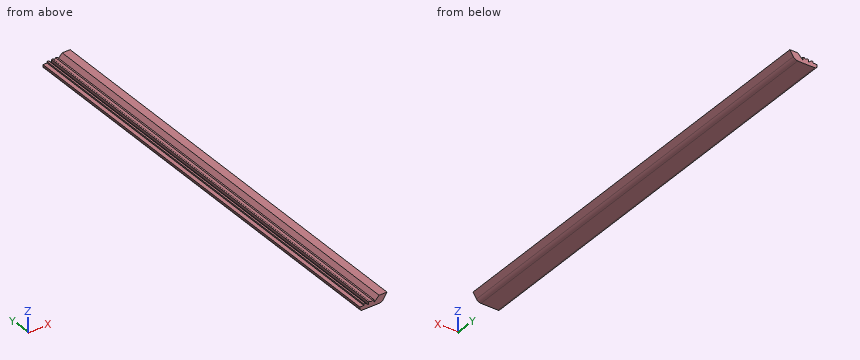
```python
from build123d import *

# Parameters (mm, degrees)
PAD_DEPTH    = 775
POCKET_DEPTH = 800


with BuildPart() as part:
    # Sketch → Pad (new body)
    with BuildSketch(Plane.XZ):
        with BuildLine():
            Line((14, -4), (-16, -4))
            ThreePointArc((-20, 0), (-18.828427, -2.828427), (-16, -4))
            Line((-20, 3), (-20, 0))
            Line((-13, 3), (-20, 3))
            Line((-13, 5.5), (-13, 3))
            Line((-10, 5.5), (-13, 5.5))
            Line((-10, 5.5), (-5, 1))
            Line((-5, 6), (-5, 1))
            Line((5, 6), (-5, 6))
            Line((5, 6), (5, 1))
            Line((14, 10), (5, 1))
            Line((28, 10), (14, 10))
            Line((21.78, 0.396373), (28, 10))
            ThreePointArc((14, -4), (18.428584, -2.754913), (21.78, 0.396373))
        make_face()
    extrude(amount=PAD_DEPTH)

    # Sketch001 (on Face16 of Pad) → Pocket (cut)
    with BuildSketch(Plane.XZ.offset(775)):
        with BuildLine():
            ThreePointArc((-2.51, 6.117451), (0, 4.67), (2.51, 6.117451))
            Line((-2.51, 6.117451), (2.51, 6.117451))
        make_face()
    extrude(amount=-POCKET_DEPTH, mode=Mode.SUBTRACT)


solid = part.part
```
Input: part model. Units: mm. Frame: model coordinates. Give positions to 0.01 mm unless a question says otherwise; leave off trailing zeros. Loops run counter-clockwise (first coordinate to the right, second up) from the corner with the lowest first, then second, coordinate; pieces in that order, holes last.
1) Contact query for flat-ended pins moving along their axis: pin 1 (0.8 mm diameter, centred on y = -278.5, z = 4.5, fed in from -X); pin 2 (3 mm diameter, centred on x = 7.5, y = -387.5, fed in from +Z); pin 3 (0.8 mm diameter, centred on x = 3.5, y = -257, fed in from +Z). Output: stop coordinate, or through.
A:
pin 1: stops at x = -13
pin 2: stops at z = 5
pin 3: stops at z = 6
2) Section query A-A on y = -462. Return the cut outline in (x, z).
A:
outline: (-20, 0) arc R4 ccw to (-16, -4) - (14, -4) arc R9.67 ccw to (21.78, 0.4) - (28, 10) - (14, 10) - (5, 1) - (5, 6) - (2.44, 6) arc R2.9 cw to (-2.44, 6) - (-5, 6) - (-5, 1) - (-10, 5.5) - (-13, 5.5) - (-13, 3) - (-20, 3) - close
3) Line query: L1, parallel to X at y = -245.5, z = 2.5; L2, parallel to X at y = -36.5, z = 5.25; L3, parallel to Z at x = 15, y = -685. Output: solid intervals per line, ascending.
A:
L1: x = -20 to -6.67, -5 to 5, 6.5 to 23.14
L2: x = -13 to -9.72, -5 to -1.74, 1.74 to 5, 9.25 to 24.92
L3: z = -3.91 to 10
